For this review, take the finished solid that the model builds, in its own axes (mm). A direction names the side the tool comes from. Give positions to 0.01 mm unless a question says otherwise; leave off trailing zeros. Write each loop counter-clockwise with the first axis right and the second up, starting at its lowest first coordinate (ties: lowest second). Pieces come first, ordered by that corner, then holes.
Q1. We need section D-D (z = 1). Write out the cut boundary in (x, y), then the cut area to 3 significant figures.
Q2. Insertion check: P1, Ø1.5, axis at y = 4, z = -10.5, coming from the -X side; P2, Ø8, axis at x = -1, z = 22.5, coming from the -Y side; P3, Ø5, axis at x = 5, z = -8.5, coming from the -Y side. Each pin has a flat end and moves straight along its axis. Give the tip position at first contact, or say it passes through.
Q3. Machinability: for faces 4 (the cylindrical face through (-1.08, 4.88, -15.49)), 5 (the cylindrical face through (-7.493, -0.33, 5.316)), 6 (the cylindrical face through (-3, 0, 22)), which of the approach directions +Z, -Z, +X, -X, +Y, -Y give a long, thin tool a straight path to every point of the face, cutting with its end or side? Answer none if there is none.
Q4. For line 1 (X direction, y = 0.25, z = 26.5); line 2 (Z direction, x = -2, y = -6.5); line 3 (Z direction, x = -4, y = -1.5), list the stretches that pass through material, from the lowest coordinate up.
Q5. We need section C-C (z = 19). Write out the cut boundary in (x, y).
Q6. Mouldability with a two-part tool opening along Z and no side actions: class faces 1 (the flat face through (5, 2, 0)), 2 (the cylindrical face through (2.58, -4.05, -14.49)), 3 (the flat face through (3.1, 1.5, 11.5)) as released by +Z, released by -Z, zero draft, split by the parting line, or undercut.
```python
from build123d import *

# Parameters (mm, degrees)
F2_SIZE  = 0.5
F3_R     = 0.1
F4_SIZE2 = 0.4019237886
F4_SIZE  = 1.5


with BuildPart() as f1:
    # F0 (on Front) → F1 (revolve)
    with BuildSketch(Plane.XZ):
        Polygon((3, 32.5), (0, 32.5), (0, -16.5), (5, -16.5), (5, -15), (4.8, -15), (4.8, -14), (5, -14), (5, 0), (7.5, 0), (7.5, 11.5), (3, 11.5), align=None)
    revolve(axis=Axis((0, 0, -4.8274807632), (0, 0, -1)))

    # F2
    f2_edges = [f1.edges().sort_by_distance(p)[0] for p in [
        (-5, 0, -16.5),
        (-3, 0, 32.5),
        (-7.5, 0, 0),
    ]]
    chamfer(f2_edges, length=F2_SIZE)

    # F3
    f3_edges = [f1.edges().sort_by_distance(p)[0] for p in [
        (-5, 0, 0),
        (-3, 0, 11.5),
    ]]
    fillet(f3_edges, radius=F3_R)

    # F4
    f4_edges = [f1.edges().sort_by_distance(p)[0] for p in [
        (-7.5, 0, 11.5),
    ]]
    f4_side = f1.faces().sort_by_distance((-7.5, 0, 6))[0]
    chamfer(f4_edges, length=F4_SIZE, length2=F4_SIZE2, reference=f4_side)


solid = f1.part
```
Computed:
1. outline: circle Ø15 at (0, 0)
1. area: 177 mm2
2. P1: stops at x = -3.8
2. P2: stops at y = -3
2. P3: stops at y = -4.33
3. face 4: -Z
3. face 5: +Z, -Z
3. face 6: +Z
4. line 1: x = -2.99 to 2.99
4. line 2: z = 0 to 11.5
4. line 3: z = -16.5 to 11.5
5. outline: circle Ø6 at (0, 0)
6. face 1: released by -Z
6. face 2: undercut
6. face 3: released by +Z
